CAD build for the part. Positions are in the model's coordinates, mm. Face numbers are marked on the shaded views. A direction names the side the tool comes from. Round coordinates to 2 decimals unless told otherwise and drop trailing zeros. Loops run counter-clockwise (first coordinate to the right, second up) from the corner with the lowest first, then second, coordinate; pieces in that order, holes last. Notation, with made-up numbers: M 3.25,84 L 7.25,84 A11 cw 7.25,103 Z; hole C 42,8 d3. An arc over 180 degrees is marked long. Put each result on its own line as item: value. Start each with the question number.
Autodesk Inventor part; units mm, degrees
ref_plane "YZ Plane" through (0, 0, 0) normal (1, 0, 0) x (0, 1, 0)
ref_plane "XZ Plane" through (0, 0, 0) normal (0, 1, 0) x (-1, 0, 0)
ref_plane "XY Plane" through (0, 0, 0) normal (0, 0, 1) x (1, 0, 0)
ref_plane "Work Plane1" through (0, 0, 0) normal (0, 0, 1) x (1, 0, 0)
sketch "Sketch1" plane through (0, 0, 0) normal (0, 0, 1) x (1, 0, 0)
  line L0 (22.5, 10) -> (22.5, -10) construction
  line L1 (-22.5, 10) -> (22.5, 10) construction
  line L2 (-22.5, -10) -> (-22.5, 10) construction
  line L3 (22.5, -10) -> (-22.5, -10) construction
  circle A0 centre (-13.1, -5.1) radius 0.75 construction
  circle A1 centre (-13.1, 5.1) radius 0.75 construction
  circle A2 centre (-2.44, 7) radius 0.5 construction
  circle A3 centre (-3.81, -8) radius 0.5 construction
  circle A4 centre (-1.27, -8) radius 0.5 construction
  circle A5 centre (1.27, -8) radius 0.5 construction
  circle A6 centre (-21.25, -8.75) radius 0.8
  circle A7 centre (21.25, -8.75) radius 0.8
  circle A8 centre (-21.25, 8.75) radius 0.8
  circle A9 centre (21.25, 8.75) radius 0.8
  circle A10 centre (3.81, -8) radius 0.5 construction
  circle A11 centre (2.44, 7) radius 0.5 construction
  circle A12 centre (13.1, 5.1) radius 0.75 construction
  circle A13 centre (13.1, -5.1) radius 0.75 construction
  circle A14 centre (-13.1789, 0.0006) radius 7.9502 construction
  circle A15 centre (13.1, 0) radius 7.9502 construction
  circle A16 centre (-21.25, 8.75) radius 3
  circle A17 centre (-21.25, -8.75) radius 3
  arc A18 (-19.216, 6.5448) -> (-19.216, -6.5448) centre (-13.1795, 0) ccw
  arc A19 (-24.0244, 9.8913) -> (-24.0244, -9.8913) centre (0.0206, 0) ccw
  line L4 (0, 10) -> (0, -10) construction
  line L5 (-6.9, -24) -> (6.9, -24) construction
  line L6 (-5.35, -25.55) -> (5.35, -25.55) construction
  line L7 (5.35, -22.45) -> (-5.35, -22.45) construction
  arc A20 (-5.35, -22.45) -> (-5.35, -25.55) centre (-5.35, -24) ccw construction
  arc A21 (5.35, -25.55) -> (5.35, -22.45) centre (5.35, -24) ccw construction
  arc A22 (-24.0244, -9.8913) -> (-13.3779, -22.2819) centre (0.0206, 0) ccw
  line L8 (-9.9794, -24) -> (9.9794, -24) construction
  line L9 (-6.8794, -27.1) -> (6.8794, -27.1)
  line L10 (6.8794, -20.9) -> (-6.8794, -20.9) construction
  arc A23 (-9.3384, -25.8877) -> (-6.8794, -27.1) centre (-6.8794, -24) ccw
  arc A24 (6.8794, -27.1) -> (6.8794, -20.9) centre (6.8794, -24) ccw construction
  circle A25 centre (-5.35, -24) radius 1.55
  circle A26 centre (5.35, -24) radius 1.55
  arc A27 (-18.4756, -7.6087) -> (0, -20) centre (0.0206, 0) ccw
  arc A28 (-9.3384, -25.8877) -> (-13.3779, -22.2819) centre (-20.8684, -34.7387) ccw
  line L11 (6.8794, -27.1) -> (-6.8794, -27.1)
  circle A29 centre (-21.25, 8.75) radius 1
  circle A30 centre (-21.25, -8.75) radius 1
  circle A31 centre (21.25, 8.75) radius 3
  circle A32 centre (21.25, -8.75) radius 3
  arc A33 (19.216, -6.5448) -> (19.216, 6.5448) centre (13.1795, 0) ccw
  arc A34 (24.0244, -9.8913) -> (24.0244, 9.8913) centre (-0.0206, 0) ccw
  arc A35 (13.3779, -22.2819) -> (24.0244, -9.8913) centre (-0.0206, 0) ccw
  arc A36 (6.8794, -27.1) -> (9.3384, -25.8877) centre (6.8794, -24) ccw
  arc A37 (0, -20) -> (18.4756, -7.6087) centre (-0.0206, 0) ccw
  arc A38 (13.3779, -22.2819) -> (9.3384, -25.8877) centre (20.8684, -34.7387) ccw
  circle A39 centre (21.25, 8.75) radius 1
  circle A40 centre (21.25, -8.75) radius 1
  point P0 (0, 0)
  point P1 (0, -24)
  point P2 (0, 0)
  point P3 (0, -24)
  point P4 (-8.2502, -26.7804)
  point P5 (22.095, 8.2152)
  point P6 (22.095, 9.2848)
  point P7 (22.095, -9.2848)
  point P8 (22.095, -8.2152)
  dimension "d0" = 6
  dimension "d11" = 17.5
  dimension "d16" = 15.9004
  dimension "d17" = 8.9036
  dimension "d19" = 8.9036
  dimension "d21" = 13.8
  dimension "d22" = 3.1
  dimension "d24" = 9.9794
  dimension "d25" = 19.9588
  dimension "d26" = 6.2
  dimension "d29" = 14.5355
  dimension "d32" = 24
  dimension "d33" = 26
  dimension "d34" = 0.2
  dimension "d37" = 0.2
extrude "Extrusion1" add sketch "Sketch1" along normal blind 3 contours A16 | A16 A18 A17 A19 | A17 | A17 A27 A37 A32 A35 A38 A36 L9 A23 A28 A22 | A32 | A33 A31 A34 A32 | A31
equation "\"d17\" = d19"
equation "\"d25\" = 2 * d24"
equation "\"d26\" = 2 * d22"
properties part number "mount" material "ABS Plastic"
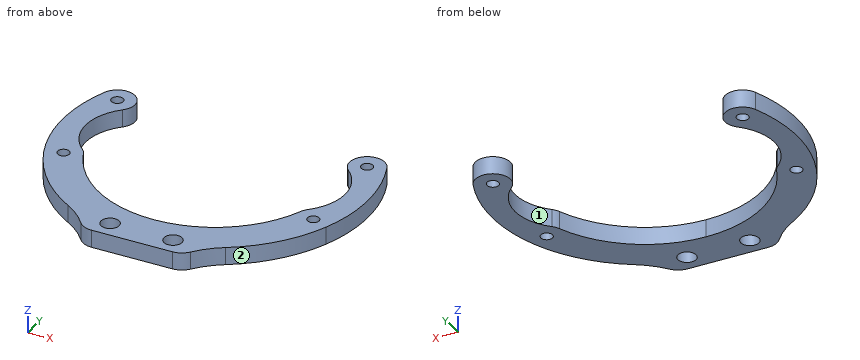
(1) Tool access for the marked faces 1 and 2: list every direction of +Z, -Z, +X, -X, +Y, -Y with a clear straight run to the whole face (end or side of a thin tool).
(2) Drill centre lines: line 1 along X through (y, z) = (9.5, 2.65); line 2 along Y through (x, z) = (-21.25, 2.05); line 3 along Y through (x, z) = (20.5, 2). Where is each one in solid material? Low to high.
(3) Cut at B-B on x = 6. List the corners of the cut face in (y, z).
(4) Flat gauge pins, fed straight in: pin 1 Ø1.5 at (y, z) = (-9, 1.5) entering from +X; pin 2 Ø3 at (x, y) = (5.35, -24) entering from +Z; pin 3 Ø1 at (y, z) = (-21, 0.5) entering from +X; pin 4 Ø1 at (x, z) = (11.5, 2) entering from +Y. Where does each tip first touch, or does it go through?
(5) Cut at A-A on y = -18.5. List the corners of the cut face in (x, z), and give its area (3 significant figures).
(6) Cut at D-D on x = 21.25. List the corners of the cut face in (y, z), and give its area (3 significant figures).
(7) Cut at C-C on z = 0.7. List the corners of the cut face in (x, y), and give its area (3 significant figures).
Taken from the geometry:
1. face 1: +Z, -Z
1. face 2: +Z, -Z, +X, -Y
2. line 1: -24.18 to -21.91, -20.59 to -18.35, 18.35 to 20.59, 21.91 to 24.18
2. line 2: -14.95 to -9.75, -7.75 to -3.76, 3.76 to 7.75, 9.75 to 11.75
2. line 3: -15.97 to -9.41, -8.09 to -5.07, 5.07 to 8.09, 9.41 to 11.65
3. outline: M -27.1,0 L -25.41,0 L -25.41,3 L -27.1,3 Z; M -22.59,0 L -19.07,0 L -19.07,3 L -22.59,3 Z
4. pin 1: x = 24.64
4. pin 2: through
4. pin 3: x = 15.97
4. pin 4: y = -15.98
5. outline: M -18.25,0 L -7.58,0 L -7.58,3 L -18.25,3 Z; M 7.58,0 L 18.25,0 L 18.25,3 L 7.58,3 Z
5. area: 64.0 mm2
6. outline: M -14.95,0 L -9.75,0 L -9.75,3 L -14.95,3 Z; M -7.75,0 L -3.76,0 L -3.76,3 L -7.75,3 Z; M 3.76,0 L 7.75,0 L 7.75,3 L 3.76,3 Z; M 9.75,0 L 11.75,0 L 11.75,3 L 9.75,3 Z
6. area: 45.5 mm2
7. outline: M -24.02,-9.89 A26 ccw -13.38,-22.28 A14.53 cw -9.34,-25.89 A3.1 ccw -6.88,-27.1 L 6.88,-27.1 A3.1 ccw 9.34,-25.89 A14.54 cw 13.38,-22.28 A26 ccw 24.02,-9.89 A26 ccw 24.02,9.89 A3 ccw long 19.22,6.54 A8.9 cw 19.22,-6.54 A3 ccw 18.48,-7.61 A20 cw 0,-20 A20 cw -18.48,-7.61 A3 ccw -19.22,-6.54 A8.9 cw -19.22,6.54 A3 ccw long -24.02,9.89 A26 ccw Z; hole C -21.25,-8.75 d2; hole C -21.25,8.75 d2; hole C -5.35,-24 d3.1; hole C 5.35,-24 d3.1; hole C 21.25,-8.75 d2; hole C 21.25,8.75 d2
7. area: 533 mm2
